```python
from build123d import *

# Parameters (mm, degrees)
SKETCH1_R           = 5.5626
BOSS_EXTRUDE1_DEPTH = 75
SKETCH5_R           = 5.5626
SKETCH5_R_2         = 5
CUT_EXTRUDE2_DEPTH  = 20
SKETCH6_R           = 5.5626
SKETCH6_R_2         = 5
CUT_EXTRUDE3_DEPTH  = 35.95


with BuildPart() as part:
    # Sketch1 → Boss-Extrude1 (new body)
    with BuildSketch(Plane.XY):
        Circle(SKETCH1_R)
    extrude(amount=BOSS_EXTRUDE1_DEPTH)

    # Sketch5 → Cut-Extrude2 (cut)
    with BuildSketch(Plane.XY.offset(20)):
        Circle(SKETCH5_R)
        Circle(SKETCH5_R_2, mode=Mode.SUBTRACT)
    extrude(amount=-CUT_EXTRUDE2_DEPTH, mode=Mode.SUBTRACT)

    # Sketch6 → Cut-Extrude3 (cut)
    with BuildSketch(Plane.XY.offset(39.05)):
        Circle(SKETCH6_R)
        Circle(SKETCH6_R_2, mode=Mode.SUBTRACT)
    extrude(amount=CUT_EXTRUDE3_DEPTH, mode=Mode.SUBTRACT)


solid = part.part
```
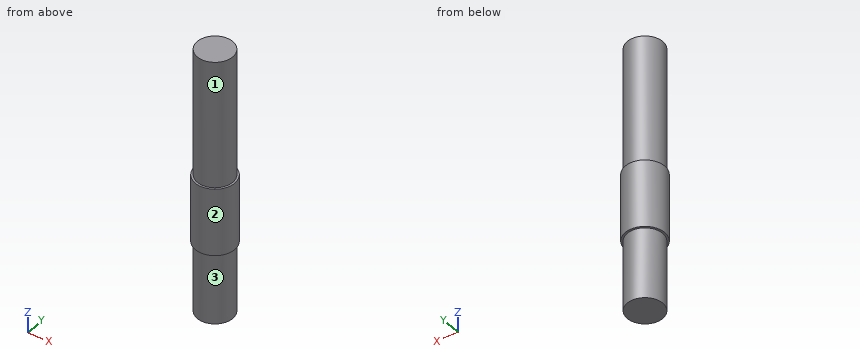
Source: CAD feature listing. Evaluate the final solid. Frame: model axes, mm. Face numbers are marked on the shaded views. A direction names the side the tool comes from. Round coordinates to 2 decimals unless told otherwise and drop trailing zeros. Loops run counter-clockwise (first coordinate to the right, second up) from the corner with the lowest first, then second, coordinate; pieces in that order, holes last. Notation, with made-up numbers: M -11.5,-34.75 L 34.5,-34.75 A12 cw 34.5,-18.75 Z; hole C -29,-33 d9. An arc over 180 degrees is marked long. Use a Markdown table: item, result. Add a question column.
1. Section query D-D on z = 12.5. Return the cut outline in (x, y).
2. Reachability of the marked faces 1, 2 and 3 from +Z, -Z, +X, -X, +Y, -Y: full face, straight path, thin tool, end or side. Return the list, or none.
3. Contact query for flat-ended pins moving along their axis: P1, Ø6, axis at y = -3.5, z = 27.5, coming from the +X side; P2, Ø1, axis at y = 3.5, z = 16, coming from the -X side; P3, Ø6, axis at x = 3, z = 63.5, coming from the -Y side. Output: stop coordinate, or through.
4. Section query C-C on z = 26. Return the cut outline in (x, y).
5. Section query A-A on x = 0. Return the cut outline in (y, z).
6. Line query: line 1 (Z direction, x = -4.25, y = -3); line 2 (Y direction, x = 0, z = 11); line 3 (Y direction, x = 2.25, z = 21). Output: solid intervals per line, ascending.
Reported:
| question | item | result |
|---|---|---|
| 1 | outline | C 0,0 d10 |
| 2 | face 1 | +Z |
| 2 | face 2 | +Z, -Z |
| 2 | face 3 | -Z |
| 3 | P1 | stops at x = 5.54 |
| 3 | P2 | stops at x = -4 |
| 3 | P3 | stops at y = -5 |
| 4 | outline | C 0,0 d11.13 |
| 5 | outline | M -5.56,20 L -5,20 L -5,0 L 5,0 L 5,20 L 5.56,20 L 5.56,39.05 L 5,39.05 L 5,75 L -5,75 L -5,39.05 L -5.56,39.05 Z |
| 6 | line 1 | z = 20 to 39.05 |
| 6 | line 2 | y = -5 to 5 |
| 6 | line 3 | y = -5.09 to 5.09 |
